Part print with two shaded views. Sizes in mm from the minimum x, y, z corner. Give positions to 0.01 mm unless a question says otherwise; leave off trailing zeros. Order: outer loops, then holes, each group sorted by start corner. A loop starts at its lowest first (then second) coordinate and runs counter-clockwise, first axis right, second up. Notation, with made-up numbers: (28.5, -0.5) -> (48.5, -0.5) arc R21 cw to (48.5, 35.5) -> close; hole circle Ø5 at (61, 15.5). An arc over 180 degrees is marked (long way). Write item = value, one per line. Start each with the question number.
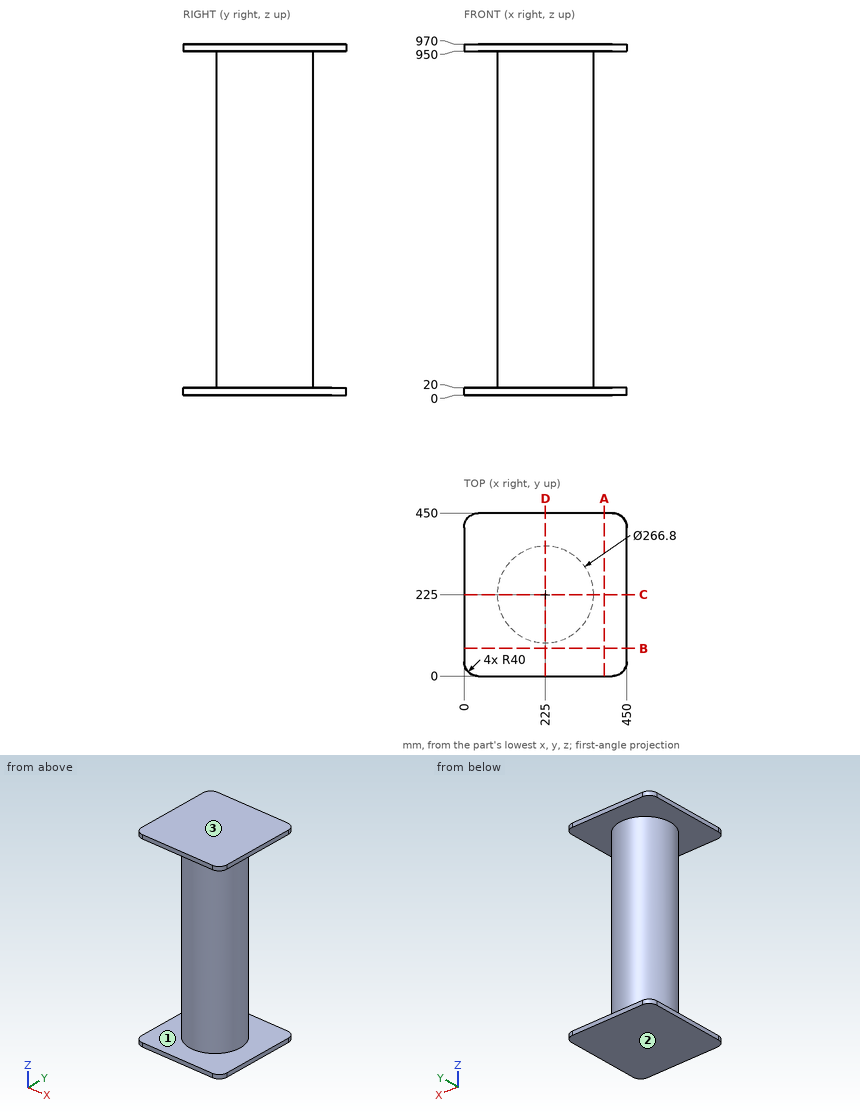
(1) Cut at C-C, the plane y = 225. Give the cut face in (x, z).
(2) Mould opens along Z. For the marked faces 1, 2 and 3 say: released by +Z, released by -Z, zero draft, split by the parting line, or undercut.
(3) Flat gauge pins, fed straight in: P1, Ø6, axis at x = 219.5, z = 354, coming from the +Y side; P2, Ø8, axis at x = 214.5, z = 529.5, coming from the -Y side; P3, Ø5, axis at y = 255, z = 312, coming from the +X side. Where does each tip first touch, or does it go through?
(4) Wall check: line 1 (Z direction, x = 159.5, y = 410); line 2 (Y direction, x = 232, z = 307.5); line 3 (Y direction, x = 311.5, z = 464.5). Give the ranges that are in metal, low to high. Write a range as [from, to].
(5) Cut at A-A, the plane x = 387.5. Give the cut face in (y, z).
Results:
q1.outline = (0, 0) -> (450, 0) -> (450, 20) -> (358.4, 20) -> (358.4, 950) -> (450, 950) -> (450, 970) -> (0, 970) -> (0, 950) -> (91.6, 950) -> (91.6, 20) -> (0, 20) -> close
q2.face_1 = undercut
q2.face_2 = released by -Z
q2.face_3 = released by +Z
q3.P1 = 358.38
q3.P2 = 91.76
q3.P3 = 355.53
q4.line_1 = [0, 20], [950, 970]
q4.line_2 = [91.78, 358.22]
q4.line_3 = [123.45, 326.55]
q5.outline = (0, 0) -> (450, 0) -> (450, 20) -> (0, 20) -> close; (0, 950) -> (450, 950) -> (450, 970) -> (0, 970) -> close
